```python
from build123d import *

# Parameters (mm, degrees)
SKETCH1_W            = 42
SKETCH1_H            = 48
SKETCH1_R            = 19.25
SKETCH1_R_2          = 2.4
BOSS_EXTRUDE1_DEPTH  = 35
SKETCH4_W            = 19
SKETCH4_H            = 5
BOSS_EXTRUDE3_DEPTH  = 35
CUT_EXTRUDE1_REACH   = 70.367
SKETCH5_R            = 2.5
BOSS_EXTRUDE4_DEPTH  = 3
CUT_EXTRUDE2_REACH   = 62.166
SKETCH7_W            = 42
SKETCH7_H            = 24
FILLET1_R            = 1
SKETCH8_W            = 80
SKETCH8_H            = 13
BOSS_EXTRUDE5_DEPTH  = 5
CUT_EXTRUDE4_REACH   = 69.543
SKETCH10_R           = 2.5
FILLET5_R            = 30
FILLET6_R            = 10
SKETCH12_W           = 38
SKETCH12_H           = 4
BOSS_EXTRUDE6_DEPTH  = 16
CUT_EXTRUDE5_REACH   = 71.116
SKETCH13_R           = 2.5
FILLET7_R            = 10
FILLET7_OF_MIRROR1_R = 10


with BuildPart() as part:
    # Sketch1 → Boss-Extrude1 (new body)
    with BuildSketch(Plane.XY):
        Rectangle(SKETCH1_W, SKETCH1_H)
        Circle(SKETCH1_R, mode=Mode.SUBTRACT)
        with Locations((-16, 18.285714286)):
            Circle(SKETCH1_R_2, mode=Mode.SUBTRACT)
        with Locations((16, 18.285714286)):
            Circle(SKETCH1_R_2, mode=Mode.SUBTRACT)
        with Locations((16, -18.285714286)):
            Circle(SKETCH1_R_2, mode=Mode.SUBTRACT)
        with Locations((-16, -18.285714286)):
            Circle(SKETCH1_R_2, mode=Mode.SUBTRACT)
    extrude(amount=-BOSS_EXTRUDE1_DEPTH)

    # Sketch4 → Boss-Extrude3 (add)
    with BuildSketch(Plane.XY):
        with Locations((-30.5, -21.5)):
            Rectangle(SKETCH4_W, SKETCH4_H)
        with Locations((30.5, -21.5)):
            Rectangle(SKETCH4_W, SKETCH4_H)
    extrude(amount=-BOSS_EXTRUDE3_DEPTH)

    # Sketch5 → Cut-Extrude1 (cut, up to next)
    with BuildSketch(Plane(origin=(0, -19, 0), x_dir=(1, 0, 0), z_dir=(0, 1, 0)), mode=Mode.PRIVATE) as cut_extrude1_sk1:
        with Locations(Location((-25, 19, 0), (0, 0, 270))):
            Circle(SKETCH5_R)
    cut_extrude1_tool1 = extrude(cut_extrude1_sk1.sketch, amount=-CUT_EXTRUDE1_REACH, mode=Mode.PRIVATE) & part.part
    # Sketch5 → Cut-Extrude1 (cut, up to next)
    with BuildSketch(Plane(origin=(0, -19, 0), x_dir=(1, 0, 0), z_dir=(0, 1, 0)), mode=Mode.PRIVATE) as cut_extrude1_sk2:
        with Locations(Location((25, 19, 0), (0, 0, 270))):
            Circle(SKETCH5_R)
    cut_extrude1_tool2 = extrude(cut_extrude1_sk2.sketch, amount=-CUT_EXTRUDE1_REACH, mode=Mode.PRIVATE) & part.part
    add(cut_extrude1_tool1.solids().sort_by_distance((-25, -19, -19))[0], mode=Mode.SUBTRACT)
    add(cut_extrude1_tool2.solids().sort_by_distance((25, -19, -19))[0], mode=Mode.SUBTRACT)

    # Sketch6 → Boss-Extrude4 (add)
    with BuildSketch(Plane(origin=(0, 0, -35), x_dir=(-1, 0, 0), z_dir=(0, 0, -1))):
        Polygon((-21, 24), (-21, -19), (-40, -19), (-40, -24), (40, -24), (40, -19), (21, -19), (21, 24), align=None)
    extrude(amount=BOSS_EXTRUDE4_DEPTH)

    # Sketch7 → Cut-Extrude2 (cut, up to next)
    with BuildSketch(Plane.XY, mode=Mode.PRIVATE) as cut_extrude2_sk1:
        with Locations((0, 12)):
            Rectangle(SKETCH7_W, SKETCH7_H)
    cut_extrude2_tool1 = extrude(cut_extrude2_sk1.sketch, amount=-CUT_EXTRUDE2_REACH, mode=Mode.PRIVATE) & part.part
    add(cut_extrude2_tool1.solids().sort_by_distance((0, 12, 0))[0], mode=Mode.SUBTRACT)

    # Fillet1
    fillet1_edges = [part.edges().sort_by_distance(p)[0] for p in [
        (19.25, 0, -17.5),
        (-19.25, 0, -17.5),
    ]]
    fillet(fillet1_edges, radius=FILLET1_R)

    # Sketch8 → Boss-Extrude5 (add)
    with BuildSketch(Plane.XZ.offset(24)):
        with Locations((0, -44.5)):
            Rectangle(SKETCH8_W, SKETCH8_H)
    extrude(amount=-BOSS_EXTRUDE5_DEPTH)

    # Sketch10 → Cut-Extrude4 (cut, up to next)
    with BuildSketch(Plane(origin=(0, -19, 0), x_dir=(1, 0, 0), z_dir=(0, 1, 0)), mode=Mode.PRIVATE) as cut_extrude4_sk1:
        with Locations(Location((-15, 43, 0), (0, 0, 180))):
            Circle(SKETCH10_R)
    cut_extrude4_tool1 = extrude(cut_extrude4_sk1.sketch, amount=-CUT_EXTRUDE4_REACH, mode=Mode.PRIVATE) & part.part
    # Sketch10 → Cut-Extrude4 (cut, up to next)
    with BuildSketch(Plane(origin=(0, -19, 0), x_dir=(1, 0, 0), z_dir=(0, 1, 0)), mode=Mode.PRIVATE) as cut_extrude4_sk2:
        with Locations(Location((15, 43, 0), (0, 0, 180))):
            Circle(SKETCH10_R)
    cut_extrude4_tool2 = extrude(cut_extrude4_sk2.sketch, amount=-CUT_EXTRUDE4_REACH, mode=Mode.PRIVATE) & part.part
    add(cut_extrude4_tool1.solids().sort_by_distance((-15, -19, -43))[0], mode=Mode.SUBTRACT)
    add(cut_extrude4_tool2.solids().sort_by_distance((15, -19, -43))[0], mode=Mode.SUBTRACT)

    # Fillet5
    fillet5_edges = [part.edges().sort_by_distance(p)[0] for p in [
        (-40, -21.5, -51),
        (40, -21.5, -51),
    ]]
    fillet(fillet5_edges, radius=FILLET5_R)

    # Fillet6
    fillet6_edges = [part.edges().sort_by_distance(p)[0] for p in [
        (-40, -21.5, 0),
        (40, -21.5, 0),
    ]]
    fillet(fillet6_edges, radius=FILLET6_R)

    # Sketch12 → Boss-Extrude6 (add)
    with BuildSketch(Plane.ZY.offset(21)):
        with Locations((-19, -2)):
            Rectangle(SKETCH12_W, SKETCH12_H)
    boss_extrude6 = extrude(amount=BOSS_EXTRUDE6_DEPTH)

    # Sketch13 → Cut-Extrude5 (cut, up to next)
    with BuildSketch(Plane(origin=(0, 0, 0), x_dir=(1, 0, 0), z_dir=(0, 1, 0)), mode=Mode.PRIVATE) as cut_extrude5_sk1:
        with Locations(Location((-29, 8, 0), (0, 0, 270))):
            Circle(SKETCH13_R)
    cut_extrude5_tool1 = extrude(cut_extrude5_sk1.sketch, amount=-CUT_EXTRUDE5_REACH, mode=Mode.PRIVATE) & part.part
    # Sketch13 → Cut-Extrude5 (cut, up to next)
    with BuildSketch(Plane(origin=(0, 0, 0), x_dir=(1, 0, 0), z_dir=(0, 1, 0)), mode=Mode.PRIVATE) as cut_extrude5_sk2:
        with Locations(Location((-29, 30, 0), (0, 0, 270))):
            Circle(SKETCH13_R)
    cut_extrude5_tool2 = extrude(cut_extrude5_sk2.sketch, amount=-CUT_EXTRUDE5_REACH, mode=Mode.PRIVATE) & part.part
    cut_extrude5_1 = cut_extrude5_tool1.solids().sort_by_distance((-29, 0, -8))[0]
    add(cut_extrude5_1, mode=Mode.SUBTRACT)
    cut_extrude5_2 = cut_extrude5_tool2.solids().sort_by_distance((-29, 0, -30))[0]
    add(cut_extrude5_2, mode=Mode.SUBTRACT)
    cut_extrude5 = cut_extrude5_1 + cut_extrude5_2  # Cut-Extrude5 as one shape, for the pattern or mirror that repeats it

    # Fillet7
    fillet7_edges = [part.edges().sort_by_distance(p)[0] for p in [
        (-37, -2, 0),
        (-37, -2, -38),
    ]]
    fillet(fillet7_edges, radius=FILLET7_R)

    # Mirror1: Boss-Extrude6, Cut-Extrude5 across plane
    add(boss_extrude6.mirror(Plane(origin=(0, 0, 0), x_dir=(0, 0, 1), z_dir=(1, 0, 0))))
    add(cut_extrude5.mirror(Plane(origin=(0, 0, 0), x_dir=(0, 0, 1), z_dir=(1, 0, 0))), mode=Mode.SUBTRACT)

    # Fillet7 of Mirror1
    fillet7_of_mirror1_edges = [part.edges().sort_by_distance(p)[0] for p in [
        (37, -2, 0),
        (37, -2, -38),
    ]]
    fillet(fillet7_of_mirror1_edges, radius=FILLET7_OF_MIRROR1_R)


solid = part.part
```
Geometry: final body of the model. Coordinates: model frame, mm. A direction names the side the tool comes from. Round coordinates to 2 decimals unless told otherwise and drop trailing zeros. Write each loop counter-clockwise with the first axis right and the second up, starting at its lowest first coordinate (ties: lowest second). Pieces come first, ordered by that corner, then holes. Notation, with made-up numbers: M -15,-16.75 L 10,-16.75 A33 ccw 10,14.25 Z; hole C 34,74.25 d6. An arc over 180 degrees is marked long. Answer in a Markdown table with one row per item. Add a question column.
(1) Contact query for flat-ended pins moving along their axis: pin 1 (3 mm diameter, centred on x = 14.5, y = -20, fed in from -Z); pin 2 (5 mm diameter, centred on y = -5.5, z = -32, fed in from -X); pin 3 (12 mm diameter, centred on y = -8.5, z = -20.5, fed in from +X); pin 4 (4 mm diameter, centred on x = 31.5, y = -7, fed in from -Z). Output: stop coordinate, or through.
(2) Cut plane B-B, the plane x = -25. Return the cut outline in (y, z), then the cut area to 3 significant figures.
(3) Cut plane D-D, the plane x = 15. Return the cut outline in (y, z).
(4) Reachability of faces 1 (the face through (-29, -4, -19)), 2 (the face through (-0.41, -19.246, -17.255)), 3 (the face through (-17.9, -19.75, -17.26)), 4 (the face through (-23.31, -21.46, -20.84)), 5 (the face through (26.52, -1.97, -30.33)) from +Z, -Z, +X, -X, +Y, -Y: full face, straight path, thin tool, end or side. Return the list, or none.
(5) Draft query along Z for faces 6 (the face through (26.52, -1.97, -8.33)), 7 (the face through (36.99, -21.46, -2.85)), 8 (the face through (-21, -12, -19)). Return one class per face: pulls with the +Z half, pulls with the -Z half, needs draft (parallel to the pull), parting line crosses it, or undercut.
(6) Cut plane C-C, the plane z = -8. Return the cut outline in (x, y), then the cut area to 3 significant figures.
(7) Cut plane A-A, the plane z = -19. Return the cut outline in (x, y).
(8) Ray query, L1, parallel to Y at x = -23.5, z = -27.5; L2, parallel to X at y = -19.5, z = -20; L3, parallel to Y at x = 27, z = -30. Return the intervals inside material, ascending.
Established:
| question | item | result |
|---|---|---|
| 1 | pin 1 | z = -50.85 |
| 1 | pin 2 | x = -36.8 |
| 1 | pin 3 | x = 37 |
| 1 | pin 4 | through |
| 2 | outline | M -24,-46.98 L -19,-46.98 L -19,-21.5 L -24,-21.5 Z; M -24,-16.5 L -19,-16.5 L -19,0 L -24,0 Z; M -4,-38 L 0,-38 L 0,0 L -4,0 Z |
| 2 | area | 362 mm² |
| 3 | outline | M -24,-50.58 L -19,-50.58 L -19,-45.5 L -24,-45.5 Z; M -24,-40.5 L -19,-40.5 L -19,-38 L 0,-38 L 0,-35 L -12.06,-35 L -12.06,0 L -16.1,0 L -16.1,-35 L -20.47,-35 L -20.47,0 L -24,0 Z |
| 4 | face 1 | +Z, -Z, -X |
| 4 | face 2 | +Z, +Y |
| 4 | face 3 | +Z |
| 4 | face 4 | -Y |
| 4 | face 5 | +Y |
| 5 | face 6 | undercut |
| 5 | face 7 | pulls with the +Z half |
| 5 | face 8 | needs draft |
| 6 | outline | M -39.8,-24 L 39.8,-24 L 39.8,-19 L 21,-19 L 21,-4 L 26.5,-4 L 26.5,0 L 20.23,0 A1 ccw 19.23,-0.95 A19.25 cw -19.23,-0.95 A1 ccw -20.23,0 L -26.5,0 L -26.5,-4 L -21,-4 L -21,-19 L -39.8,-19 Z; M -36.8,-4 L -31.5,-4 L -31.5,0 L -36.8,0 Z; M 31.5,-4 L 36.8,-4 L 36.8,0 L 31.5,0 Z; hole C -16,-18.29 d4.8; hole C 16,-18.29 d4.8 |
| 6 | area | 664 mm² |
| 7 | outline | M -40,-24 L -27.5,-24 L -27.5,-19 L -40,-19 Z; M -37,-4 L -21,-4 L -21,-19 L -22.5,-19 L -22.5,-24 L 22.5,-24 L 22.5,-19 L 21,-19 L 21,-4 L 37,-4 L 37,0 L 20.23,0 A1 ccw 19.23,-0.95 A19.25 cw -19.23,-0.95 A1 ccw -20.23,0 L -37,0 Z; M 27.5,-24 L 40,-24 L 40,-19 L 27.5,-19 Z; hole C -16,-18.29 d4.8; hole C 16,-18.29 d4.8 |
| 8 | L1 | -24 to -19, -4 to 0 |
| 8 | L2 | -40 to -27.29, -22.71 to -18.07, -13.93 to 13.93, 18.07 to 22.71, 27.29 to 40 |
| 8 | L3 | -24 to -19 |
